Geometry check sheet. Reference: the model listing, model coordinates, mm. Face numbers are marked on the shaded views. Give positions to 0.01 mm unless a question says otherwise; leave off trailing zeros. Write each loop counter-clockwise with the first axis right and the second up, starting at its lowest first coordinate (ties: lowest second). Pieces come first, ordered by that corner, then holes.
(1) Cross-section at B-B (y = 27). Record the boundary of the cut face in (x, z) (3 decimals), and give its area (3 significant figures).
(2) Thickness scan on line 1 along Z through (x, y) = (-1, 14); line 2 along X through (y, z) = (1.5, 0); line 3 along X through (y, z) = (34, 0) (3 decimals). Record the ranges inside material, lowest first.
(3) Cross-section at A-A (z = 0). Record the boundary of the cut face in (x, y) (3 decimals), and give its area (3 significant figures).
(4) Mould release check, pull along Z, two halves, no side actions. Record for the marked faces 1, 2 and 3: +Z half, -Z half, draft (parallel to the pull), parting line (faces both ways), or undercut.
(5) Depth check by flat-ended pin: P1, Ø5, axis at x = 6, y = 91.5, coming from the +Z side; P2, Ø1, axis at x = 37, z = 44.5, coming from the +Y side; P3, Ø1, axis at y = 83, z = -23, coming from the +X side. Enter the tip coordinate at first touch or a pass-through.
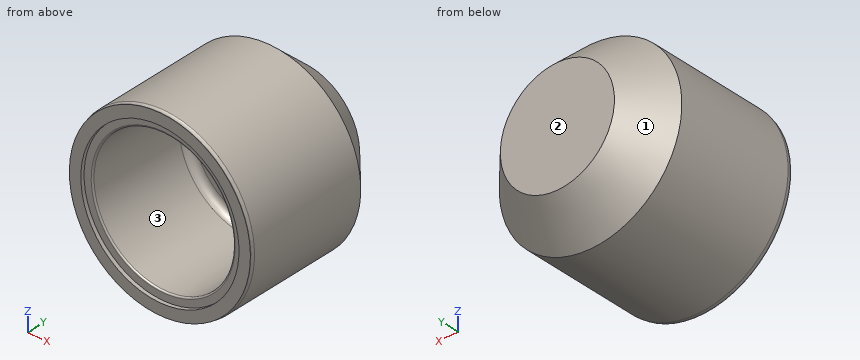
```python
from build123d import *

# Parameters (mm, degrees)
SKETCH1_R           = 59.5
SKETCH1_R_2         = 52
BOSS_EXTRUDE1_DEPTH = 2.5
SKETCH2_R           = 60
SKETCH2_R_2         = 46.365
BOSS_EXTRUDE2_DEPTH = 70
SKETCH3_R           = 60
BOSS_EXTRUDE3_DEPTH = 10
FILLET1_R           = 1
SKETCH4_R           = 37.5
FILLET2_R           = 5
FILLET3_R           = 5


with BuildPart() as part:
    # Sketch1 → Boss-Extrude1 (new body)
    with BuildSketch(Plane(origin=(0, 0, 0), x_dir=(1, 0, 0), z_dir=(0, 1, 0))):
        with Locations(Location((0, 0, 0), (0, 0, 270))):
            Circle(SKETCH1_R)
        with Locations(Location((0, 0, 0), (0, 0, 270))):
            Circle(SKETCH1_R_2, mode=Mode.SUBTRACT)
    extrude(amount=BOSS_EXTRUDE1_DEPTH)

    # Sketch2 → Boss-Extrude2 (add)
    with BuildSketch(Plane(origin=(0, 2.5, 0), x_dir=(1, 0, 0), z_dir=(0, 1, 0))):
        with Locations(Location((0, 0, 0), (0, 0, 270))):
            Circle(SKETCH2_R)
        with Locations(Location((0, 0, 0), (0, 0, 270))):
            Circle(SKETCH2_R_2, mode=Mode.SUBTRACT)
    extrude(amount=BOSS_EXTRUDE2_DEPTH)

    # Sketch3 → Boss-Extrude3 (add)
    with BuildSketch(Plane(origin=(0, 72.5, 0), x_dir=(1, 0, 0), z_dir=(0, 1, 0))):
        with Locations(Location((0, 0, 0), (0, 0, 270))):
            Circle(SKETCH3_R)
    extrude(amount=BOSS_EXTRUDE3_DEPTH)

    # Fillet1
    fillet1_edges = [part.edges().sort_by_distance(p)[0] for p in [
        (0, 2.5, -46.365),
    ]]
    fillet(fillet1_edges, radius=FILLET1_R)

    # Sketch4 → section 1 of loft1
    with BuildSketch(Plane(origin=(0, 107.5, 0), x_dir=(1, 0, 0), z_dir=(0, 1, 0)), mode=Mode.PRIVATE) as loft1_s1:
        Circle(SKETCH4_R)
    # loft up to a face of the part (loft1)
    loft([Face(Wire([part.edges().sort_by_distance((43.738117645, 82.5, -41.072826356))[0]])), loft1_s1.sketch])

    # Fillet2
    fillet2_edges = [part.edges().sort_by_distance(p)[0] for p in [
        (0, 72.5, -46.365),
    ]]
    fillet(fillet2_edges, radius=FILLET2_R)

    # Fillet3
    # the kernel refuses this fillet: 5 mm, written as the material it adds along each edge
    with BuildSketch(Plane(origin=(0, 2.5, 0), x_dir=(0, 0, 1), z_dir=(-1, 0, 0))) as fillet3_piece_1:
        with BuildLine():
            CenterArc((64.5, -2.179449472), FILLET3_R, 154.158067237, 25.841932763)
            Line((60, 0), (59.5, 0))
            Line((59.5, 0), (59.5, -2.179449472))
        make_face()
    revolve(axis=Axis((0, 2.5, 0), (0, 1, 0)))


solid = part.part
```
Reply:
1. outline: circle Ø120 at (0, 0); hole circle Ø92.73 at (0, 0)
1. area: 4,560 mm2
2. line 1: z = -59.99 to -46.35, 46.35 to 59.99
2. line 2: x = -59.64 to -52, 52 to 59.64
2. line 3: x = -60 to -46.365, 46.365 to 60
3. outline: (-60, 2.5) arc R5 cw to (-59.5, 0.321) - (-59.5, 0) - (-52, 0) - (-52, 2.5) - (-47.365, 2.5) arc R1 ccw to (-46.365, 3.5) - (-46.365, 67.5) arc R5 cw to (-41.365, 72.5) - (41.365, 72.5) arc R5 cw to (46.365, 67.5) - (46.365, 3.5) arc R1 ccw to (47.365, 2.5) - (52, 2.5) - (52, 0) - (59.5, 0) - (59.5, 0.321) arc R5 cw to (60, 2.5) - (60, 82.5) - (37.5, 107.5) - (-37.5, 107.5) - (-60, 82.5) - close
3. area: 5,590 mm2
4. face 1: parting line
4. face 2: draft
4. face 3: undercut
5. P1: stops at z = 53.83
5. P2: stops at y = 85.42
5. P3: stops at x = 55.46
